Geometry check sheet. Reference: the model listing, model coordinates, mm. A direction names the side the tool comes from. Round coordinates to 2 decimals unless told otherwise and drop trailing zeros. Order: outer loops, then holes, each group sorted by start corner. A loop starts at its lowest first (then second) coordinate and runs counter-clockwise, first axis right, second up.
(1) Thickness scan on L1, parallel to Z at x = 0, y = 4; L2, parallel to Y at x = -7.75, z = 8.75; L3, parallel to Y at x = 5.25, z = -0.5. Record the ranges inside material, lowest first.
(2) Gauge pin test, flat ends, axial feed: P1, Ø0.8, axis at y = 0.5, z = 15.5, coming from the -X side; P2, Ø12, axis at x = -2.5, z = 16, coming from the -Y side; P3, Ø0.8, axis at y = 1, z = 17, coming from the +X side. Record the tip position at first contact, or that the pin passes through.
(3) Cross-section at B-B on y = -0.75. Enter the section's corners in (x, z).
(4) Cross-section at C-C on y = 15. Enter the section's corners in (x, z), and give its area (3 significant figures).
(5) Draft check along X on faces 5 (the face through (0, -5, 0)), 6 (the face through (-1.08, 6.95, -4.88)), 7 (the face through (3, 1, 14)). Enter one of: pulls with the +X half, pulls with the -X half, needs draft (parallel to the pull), parting line crosses it, or undercut.
(6) Set-up check for faces 1 (the face through (-3, 15, 0)), 2 (the face through (8, 1, 14)), 3 (the face through (-1.302, -1.823, -9.915)), 4 (the face through (-2, 1, 14)): record each of +Z, -Z, +X, -X, +Y, -Y from which the full face is reachable in a straight line by a thin tool's end or side.
(7) Cross-section at A-A on z = 14.75. Enter the section's corners in (x, y), and give its area (3 significant figures).
Autodesk Inventor part; units mm, degrees
ref_plane "YZ Plane" through (0, 0, 0) normal (1, 0, 0) x (0, 1, 0)
ref_plane "XZ Plane" through (0, 0, 0) normal (0, 1, 0) x (-1, 0, 0)
ref_plane "XY Plane" through (0, 0, 0) normal (0, 0, 1) x (1, 0, 0)
sketch "Sketch1" plane through (0, 0, 0) normal (0, 1, 0) x (-1, 0, 0)
  circle A0 centre (0, 0) radius 10
  line L0 (10, 0) -> (-10, 0)
  line L1 (-10, 0) -> (-10, 14)
  line L2 (-10, 14) -> (10, 14)
  line L3 (10, 14) -> (10, 0)
  line L4 (-5.5, 14) -> (-4.5, 14)
  line L5 (-0.5, 14) -> (0.5, 14)
  line L6 (4.5, 14) -> (5.5, 14)
  line L7 (5.5, 14) -> (4.5, 14)
  line L8 (4.5, 14) -> (4.5, 19)
  line L9 (4.5, 19) -> (5.5, 19)
  line L10 (5.5, 19) -> (5.5, 14)
  line L11 (0.5, 14) -> (-0.5, 14)
  line L12 (-0.5, 14) -> (-0.5, 19)
  line L13 (-0.5, 19) -> (0.5, 19)
  line L14 (0.5, 19) -> (0.5, 14)
  line L15 (-4.5, 14) -> (-5.5, 14)
  line L16 (-5.5, 14) -> (-5.5, 19)
  line L17 (-5.5, 19) -> (-4.5, 19)
  line L18 (-4.5, 19) -> (-4.5, 14)
  point P0 (0, 14)
  point P1 (5, 14)
  point P2 (-5, 14)
  dimension "d0" = 20
  dimension "d1" = 20
  dimension "d2" = 14
  dimension "d5" = 1
  dimension "d6" = 1
  dimension "d7" = 1
  dimension "d8" = 5
  dimension "d9" = 5
  dimension "d10" = 5
extrude "Extrusion1" add sketch "Sketch1" along normal blind 1.5
sketch "Sketch2" plane through (0, 0, 0) normal (0, -1, 0) x (1, 0, 0)
  circle A0 centre (0, 0) radius 10
extrude "Extrusion2" add sketch "Sketch2" along normal blind 5
sketch "Sketch3" plane through (0, 1.5, 0) normal (0, 1, 0) x (1, 0, 0)
  circle A0 centre (0, 0) radius 6.5
  dimension "d13" = 13
extrude "Extrusion3" add sketch "Sketch3" along normal blind 2
sketch "Sketch4" plane through (0, 3.5, 0) normal (0, 1, 0) x (1, 0, 0)
  circle A0 centre (0, 0) radius 5
  dimension "d16" = 10
extrude "Extrusion4" add sketch "Sketch4" along normal blind 7
thread "Thread1"
sketch "Sketch5" plane through (0, 10.5, 0) normal (0, 1, 0) x (1, 0, 0)
  circle A0 centre (0, 0) radius 3
  line L0 (0, 0) -> (1.5, 0)
  line L1 (1.5, -2.5981) -> (1.5, 2.5981)
  point P0 (0.0162, 1.5)
  point P1 (-2.4, 1.8)
  dimension "d21" = 6
  dimension "d27" = 1.5
extrude "Extrusion5" add sketch "Sketch5" along normal blind 10
fillet "Fillet1" radius 1 1 edges at (-10, -5, 0)
fillet "Fillet2" radius 0.2 6 edges at (5.5, 0.75, 19) (4.5, 0.75, 19) (0.5, 0.75, 19) (-0.5, 0.75, 19) (-4.5, 0.75, 19) (-5.5, 0.75, 19)
properties part number "PotMeter"
Found:
1. L1: z = -5 to 5
1. L2: y = 0 to 1.5
1. L3: y = -5 to 3.5
2. P1: stops at x = -5.5
2. P2: stops at y = 0
2. P3: stops at x = 5.5
3. outline: circle Ø20 at (0, 0)
4. outline: circle Ø6 at (0, 0)
4. area: 28.3 mm2
5. face 5: needs draft
5. face 6: parting line crosses it
5. face 7: undercut
6. face 1: +Y
6. face 2: +Z, +X, +Y, -Y
6. face 3: -Y
6. face 4: +Z, +Y, -Y
7. outline: (-5.5, 0) - (-4.5, 0) - (-4.5, 1.5) - (-5.5, 1.5) - close; (-0.5, 0) - (0.5, 0) - (0.5, 1.5) - (-0.5, 1.5) - close; (4.5, 0) - (5.5, 0) - (5.5, 1.5) - (4.5, 1.5) - close
7. area: 4.50 mm2
